CAD build for the part. Positions are in the model's coordinates, mm. Round coordinates to 2 decimals unless told otherwise and drop trailing zeros. Write each loop counter-clockwise with the first axis right and the second up, starting at its lowest first coordinate (ties: lowest second). Pieces come first, ordered by that corner, then holes. Notation, with made-up numbers: (-31.5, -22.75) - (-21.5, -22.75) arc R15 cw to (-21.5, -6.75) - close; hole circle Ø2 at (-19.5, -4). An arc over 180 degrees is marked (long way). Put each result on its own line as item: value. Start each with the question number.
Item 1: Pin check, flat tips, straight feed: pin 1 Ø2.5 at (y, z) = (167, -20.5) entering from -X; pin 2 Ø4 at (x, y) = (-1, 164) entering from +Z; pin 3 Ø1 at (x, z) = (11.5, -3) entering from -Y; pin 4 Ø2.5 at (y, z) = (164, -20.5) entering from +X. Stop position of each tip, or through.
Item 2: Cut at D-D (x = 8). Give the cut face in (y, z), and give its area (4 significant figures).
Item 3: Cut at B-B (z = 19.5). Give the cut face in (x, y).
Item 4: Drill centre line: line 1 (Y direction, x = 8, z = -11.5). Where is it in solid material? Low to high. Write a range as from..to.
Item 5: Cut at A-A (x = 19). Give the cut face in (y, z).
Item 6: Cut at C-C (x = -1.5). Give the cut face in (y, z).
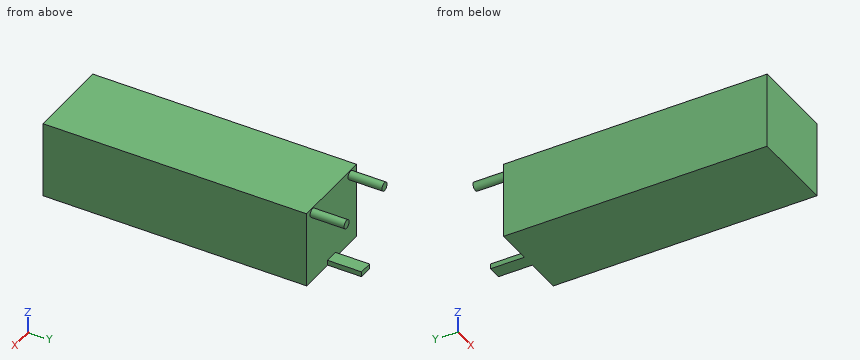
```python
from build123d import *

# Parameters (mm, degrees)
SKETCH_1_W      = 50
SKETCH_1_H      = 45
EXTRUDE_1_DEPTH = 155
SKETCH_2_R      = 2.5
SKETCH_2_W      = 8
SKETCH_2_H      = 3
EXTRUDE_2_DEPTH = 20


with BuildPart() as part:
    # 草图1 → 凸台-拉伸1 (new body)
    with BuildSketch(Plane(origin=(0, 0, 0), x_dir=(1, 0, 0), z_dir=(0, 1, 0))):
        Rectangle(SKETCH_1_W, SKETCH_1_H)
    extrude(amount=EXTRUDE_1_DEPTH)

    # 草图2 → 凸台-拉伸2 (add)
    with BuildSketch(Plane(origin=(0, 155, 0), x_dir=(1, 0, 0), z_dir=(0, 1, 0))):
        with Locations(Location((-19, -19.5, 0), (0, 0, 90))):
            Circle(SKETCH_2_R)
        with Locations(Location((19, -19.5, 0), (0, 0, 90))):
            Circle(SKETCH_2_R)
        with Locations((0, 21)):
            Rectangle(SKETCH_2_W, SKETCH_2_H)
    extrude(amount=EXTRUDE_2_DEPTH)


solid = part.part
```
Output values:
1. pin 1: x = -4
1. pin 2: z = -19.5
1. pin 3: y = 0
1. pin 4: x = 4
2. outline: (0, -22.5) - (155, -22.5) - (155, 22.5) - (0, 22.5) - close
2. area: 6,975 mm2
3. outline: (-25, 0) - (25, 0) - (25, 155) - (21.5, 155) - (21.5, 175) - (16.5, 175) - (16.5, 155) - (-16.5, 155) - (-16.5, 175) - (-21.5, 175) - (-21.5, 155) - (-25, 155) - close
4. line 1: 0..155
5. outline: (0, -22.5) - (155, -22.5) - (155, 17) - (175, 17) - (175, 22) - (155, 22) - (155, 22.5) - (0, 22.5) - close
6. outline: (0, -22.5) - (175, -22.5) - (175, -19.5) - (155, -19.5) - (155, 22.5) - (0, 22.5) - close
